Autodesk Inventor part; units mm, degrees
ref_plane "Plan de construction1" through (-13, -9.5, -10) normal (0, 0, -1) x (0, 1, 0)
ref_plane "YZ Plane" through (0, 0, 0) normal (1, 0, 0) x (0, 1, 0)
ref_plane "XZ Plane" through (0, 0, 0) normal (0, 1, 0) x (-1, 0, 0)
sketch "Esquisse1" plane through (0, 0, 0) normal (0, 0, 1) x (1, 0, 0)
  circle A0 centre (-3.5, 0) radius 2.5
  circle A1 centre (-3.5, 0) radius 2.5
  point P0 (0, 0)
ref_plane "Plan de construction1" through (-13, -9.5, -10) normal (0, 0, -1) x (0, 1, 0)
extrude "Extrusion1" add sketch "Esquisse1" against normal up to surface (10 mm away)
ref_plane "Plan de construction2" through (-3.5, 0, -9.5) normal (0, 0, -1) x (-1, 0, 0)
sketch "Esquisse2" plane through (-3.5, 0, -9.5) normal (0, 0, -1) x (-1, 0, 0)
  circle A0 centre (0, 0) radius 2.5
  circle A1 centre (0, 0) radius 2.2333
  point P0 (-3.5, 0)
extrude "Extrusion2" cut sketch "Esquisse2" along normal mid plane 0.5
sketch "Esquisxse8" plane through (-3.5, 0, 0) normal (0, 0, 1) x (1, 0, 0)
  circle A0 centre (-1.0139, -37.4629) radius 12
  circle A1 centre (-6.8791, -30.6366) radius 1.5
  circle A2 centre (-3.9931, -45.9556) radius 1.5
  circle A3 centre (7.8305, -35.7967) radius 1.5
  circle A4 centre (0, 0) radius 2.5
  arc A5 (6, 0) -> (-6, 0) centre (0, 0) ccw
  arc A6 (-12.7687, -35.0496) -> (10.3163, -33.5099) centre (-1.0139, -37.4629) ccw
  circle A7 centre (-3.9931, -45.9556) radius 1.5
  circle A8 centre (-6.8791, -30.6366) radius 1.5
  circle A9 centre (7.8305, -35.7967) radius 1.5
  line L0 (10.9482, -38.4158) -> (6, 0)
  line L1 (-6, 0) -> (-12.8221, -35.3258)
  point P0 (3.5, 0)
  dimension "d15" = 12
extrude "Extrusion6" add sketch "Esquisxse8" along normal blind 3 contours L0 A0 | A0 L1 A5 L0 picked at (-1.038, -37.5266)
sketch "Esquisse9" plane through (-3.5, 0, 3) normal (0, 0, 1) x (1, 0, 0)
  circle A0 centre (0, 0) radius 2.5
  circle A1 centre (0, 0) radius 2.5
  point P0 (3.5, 0)
extrude "Extrusion7" add sketch "Esquisse9" against normal blind 10
properties part number "bras_codeur"
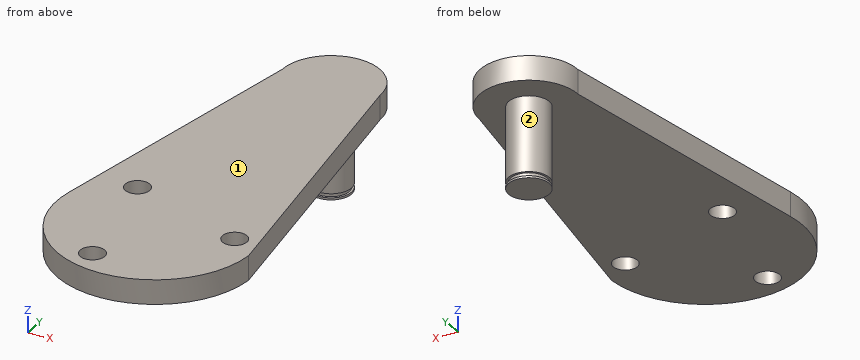
Source: CAD feature listing. Evaluate the final solid. Frame: model axes, mm. Face numbers are marked on the shaded views. A direction names the side the tool comes from. Round coordinates to 2 decimals unless told otherwise and drop trailing zeros. Loops run counter-clockwise (first coordinate to the right, second up) from the corner with the lowest first, then second, coordinate; pieces in that order, holes last. Notation, with made-up numbers: (-12.75, 10.25) - (-6.75, 10.25) arc R14 ccw to (-6.75, 34.25) - close; hole circle Ø2 at (86.25, 74.5). An arc over 180 degrees is marked (long way). Write item = value, one per line. Start each with the question number.
(1) Ray query, line 1 along Z through (x, y) = (2.5, -1.5); line 2 along Y through (x, z) = (-1.5, -2.75); line 3 along X through (y, z) = (-21.5, 0.5). Return the intervals inside material, ascending. Write a range as from..to.
(2) Section query C-C, the plane z = 0.5. Output: boundary loops of the cut face in (x, y), plus the area to 3 significant figures.
(3) Pin query (flat end, axial travel): pin 1 (5 mm diameter, centred on x = -4, z = 1.5, fed in from +Y); pin 2 (4 mm diameter, centred on x = -10.38, y = -30.64, fed in from -Z); pin 3 (5 mm diameter, centred on y = -2.5, z = -4.5, fed in from +X); pin 4 (3 mm diameter, centred on y = -42, z = 0.5, fed in from +X). Return the tip coordinate at first contact, or that it passes through.
(4) Set-up query: the marked faces 1 and 2. Return all of +Z, -Z, +X, -X, +Y, -Y with unobstructed straight access to the full face (end or side cutting, diameter ignored); none if empty.
(5) Section query A-A, the plane x = -6.75. Output: boundary loops of the cut face in (y, z), plus the area to 3 significant figures.
(6) Section query D-D, the plane z = -5.25. Output: boundary loops of the cut face in (x, y), plus the area to 3 significant figures.
(7) Section query B-B, the plane x = -3.5. Output: boundary loops of the cut face in (y, z), plus the area to 3 significant figures.
Conclusion:
q1.line_1 = 0..3
q1.line_2 = -1.5..1.5
q1.line_3 = -13.65..5.27
q2.outline = (-16.27, -35.05) arc R12 ccw (long way) to (7.45, -38.42) - (2.5, 0) arc R6 ccw to (-9.5, 0) - close; hole circle Ø3 at (-10.38, -30.64); hole circle Ø3 at (-7.49, -45.96); hole circle Ø3 at (4.33, -35.8)
q2.area = 937 mm2
q3.pin_1 = 6
q3.pin_2 = 0
q3.pin_3 = -1
q3.pin_4 = 7.1
q4.face_1 = +Z, +X, -X, +Y, -Y
q4.face_2 = -Z
q5.outline = (-49.25, 0) - (-47.26, 0) - (-47.26, 3) - (-49.25, 3) - close; (-44.65, 0) - (5.04, 0) - (5.04, 3) - (-44.65, 3) - close
q5.area = 155 mm2
q6.outline = circle Ø5 at (-3.5, 0)
q6.area = 19.6 mm2
q7.outline = (-49.42, 0) - (-2.5, 0) - (-2.5, -9.25) - (-2.23, -9.25) - (-2.23, -9.75) - (-2.5, -9.75) - (-2.5, -10) - (2.5, -10) - (2.5, -9.75) - (2.23, -9.75) - (2.23, -9.25) - (2.5, -9.25) - (2.5, 0) - (6, 0) - (6, 3) - (-49.42, 3) - close
q7.area = 216 mm2
